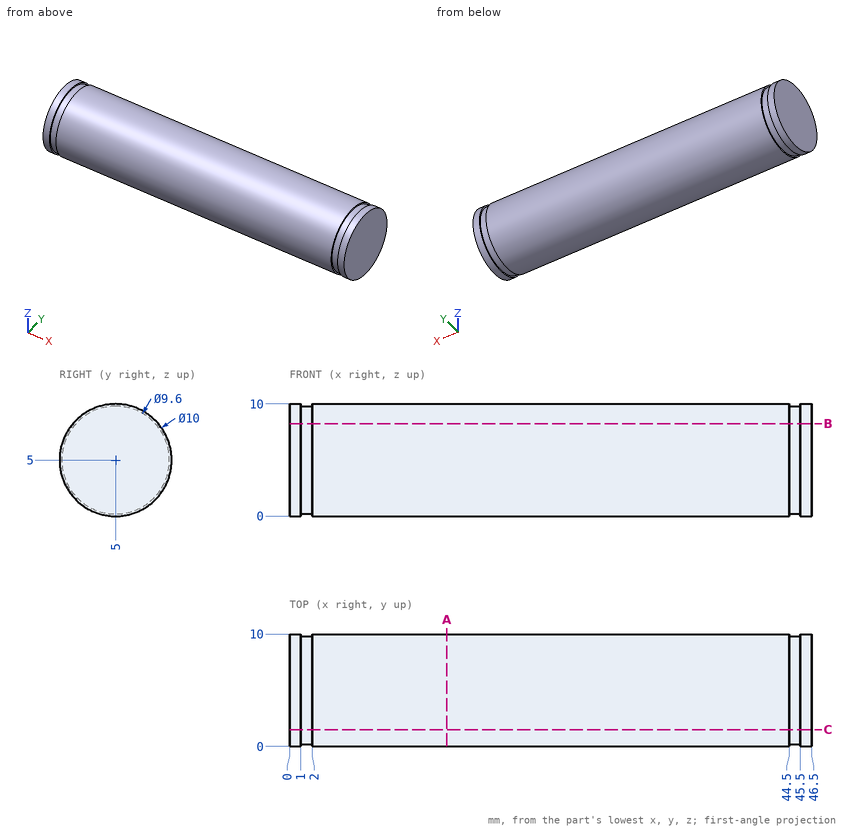
Could you check a few things on this drawing? It's one solid part, dimensions in mm from its lowest x, y, z. Give positions to 0.01 mm unless a question says otherwise; leave off trailing zeros. Loops run counter-clockwise (first coordinate to the right, second up) from the corner with the lowest first, then second, coordinate; pieces in that order, holes last. Notation, with made-up numbers: M -1.75,-19.5 L 26.25,-19.5 A25 cw 26.25,3.5 Z; hole C -36.5,-2.5 d5. An arc over 180 degrees is marked long. One line per question, with ' | ' between items. Start each with the question number.
Q1. For pin 1 Ø3 at (x, y) = (39, 2) entering from +Z; pin 2 Ø1.5 at (x, y) = (35.5, 2) entering from +Z, each with a flat end and sliding along its axis, tell me the tip position at first contact or that it passes through.
Q2. If we section it at C-C (y = 1.5): Please give me the cut outline in (x, z).
Q3. If we section it at A-A (x = 14): Please give me the cut outline in (y, z), plus the area to 3 significant figures.
Q4. If we section it at B-B (z = 8.25): Please give me the cut outline in (x, y).
Q5. If I drill on line 1 (X direction, y = 9.5, z = 3); line 2 (Y direction, x = 8.5, z = 4.75); line 3 (Z direction, x = 28.5, y = 4), over which ranges is the centre line in solid material (lowest first)? Write a range as from..to.
Computed:
1) pin 1: stops at z = 9.77 | pin 2: stops at z = 9.47
2) outline: M 0,1.43 L 1,1.43 L 1,1.72 L 2,1.72 L 2,1.43 L 44.5,1.43 L 44.5,1.72 L 45.5,1.72 L 45.5,1.43 L 46.5,1.43 L 46.5,8.57 L 45.5,8.57 L 45.5,8.28 L 44.5,8.28 L 44.5,8.57 L 2,8.57 L 2,8.28 L 1,8.28 L 1,8.57 L 0,8.57 Z
3) outline: C 5,5 d10 | area: 78.5 mm²
4) outline: M 0,1.2 L 1,1.2 L 1,1.47 L 2,1.47 L 2,1.2 L 44.5,1.2 L 44.5,1.47 L 45.5,1.47 L 45.5,1.2 L 46.5,1.2 L 46.5,8.8 L 45.5,8.8 L 45.5,8.53 L 44.5,8.53 L 44.5,8.8 L 2,8.8 L 2,8.53 L 1,8.53 L 1,8.8 L 0,8.8 Z
5) line 1: x = 0..1, 2..44.5, 45.5..46.5 | line 2: y = 0.01..9.99 | line 3: z = 0.1..9.9
